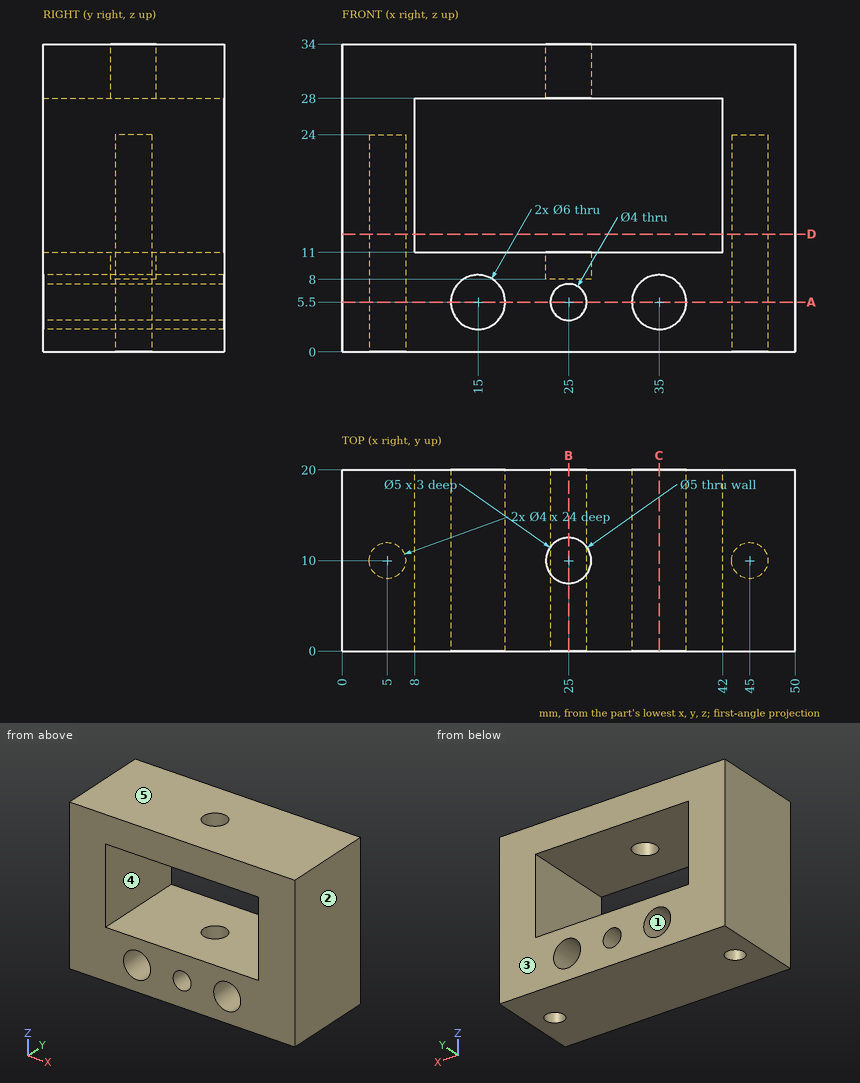
Drawing for the job (mm, zero at the part's lowest x, y, z). A direction names the side the tool comes from. Coordinates: 2 decimals unless noted, no trailing zeros. Write each loop counter-clockwise with the first axis right and the second up, starting at its lowest first coordinate (ties: lowest second). Pieces come first, ordered by that corner, then holes. Notation, with made-up numbers: (5.25, -9.5) - (27.25, -9.5) arc R34 cw to (27.25, 28.5) - close; hole circle Ø3 at (22, -22). An arc over 180 degrees is marked (long way). Write each question's results on one line, items separated by ' | '. Start each with the question number.
1) Cut at A-A (z = 5.5). Write the cut outline in (x, y), then the cut area to 3 significant figures.
2) Probe line 1 along Z through (x, y) = (35, 6.5); line 2 along Z through (x, y) = (20, 14.75); line 3 along X through (y, z) = (16, 19.5). List the from-to ranges inside material, lowest first. Write a range as from..to.
3) Flat gauge pins, fed straight in: P1, Ø8, axis at x = 15, z = 5.5, coming from the +Y side; P2, Ø3, axis at x = 25, y = 10, coming from the +Z side; P3, Ø1.2, axis at x = 5.5, y = 10, coming from the -Z side. Where does each tip first touch, or does it go through?
4) Mould opens along X. For the marked faces 1, 2 and 3 say: pulls with the +X half, pulls with the -X half, needs draft (parallel to the pull), parting line crosses it, or undercut.
5) 3-axis set-ups, long thin cutter, end or side, ignore diameter. For the marked faces 4 and 5: which of +Z, -Z, +X, -X, +Y, -Y reach the whole face in a straight line?
6) Cut at C-C (x = 35). Write the cut outline in (y, z), then the cut area to 3 significant figures.
7) Cut at D-D (z = 13). Write the cut outline in (x, y), then the cut area to 3 significant figures.
8) Cut at B-B (x = 25). Write the cut outline in (y, z), then the cut area to 3 significant figures.
Returned:
1) outline: (0, 0) - (12, 0) - (12, 20) - (0, 20) - close; (18, 0) - (23, 0) - (23, 20) - (18, 20) - close; (27, 0) - (32, 0) - (32, 20) - (27, 20) - close; (38, 0) - (50, 0) - (50, 20) - (38, 20) - close; hole circle Ø4 at (5, 10); hole circle Ø4 at (45, 10) | area: 655 mm^2
2) line 1: 0..2.5, 8.5..11, 28..34 | line 2: 0..11, 28..34 | line 3: 0..8, 42..50
3) P1: y = 20 | P2: z = 8 | P3: z = 24
4) face 1: undercut | face 2: pulls with the +X half | face 3: needs draft
5) face 4: +Y, -Y | face 5: +Z, +X, -X, +Y, -Y
6) outline: (0, 0) - (20, 0) - (20, 2.5) - (0, 2.5) - close; (0, 8.5) - (20, 8.5) - (20, 11) - (0, 11) - close; (0, 28) - (20, 28) - (20, 34) - (0, 34) - close | area: 220 mm^2
7) outline: (0, 0) - (8, 0) - (8, 20) - (0, 20) - close; (42, 0) - (50, 0) - (50, 20) - (42, 20) - close; hole circle Ø4 at (5, 10); hole circle Ø4 at (45, 10) | area: 295 mm^2
8) outline: (0, 0) - (20, 0) - (20, 3.5) - (0, 3.5) - close; (0, 7.5) - (20, 7.5) - (20, 11) - (12.5, 11) - (12.5, 8) - (7.5, 8) - (7.5, 11) - (0, 11) - close; (0, 28) - (7.5, 28) - (7.5, 34) - (0, 34) - close; (12.5, 28) - (20, 28) - (20, 34) - (12.5, 34) - close | area: 215 mm^2
